Check sheet for the drawn part. Datum: minimum x, y, z corner. Units: mm. A direction names the side the tool comes from. Give positions to 0.01 mm unless a question says otherwise; leave off trailing zeros. Order: outer loops, then holes, each group sorted by start corner. A loop starts at its lowest first (then second) coordinate and runs counter-clockwise, first axis right, second up.
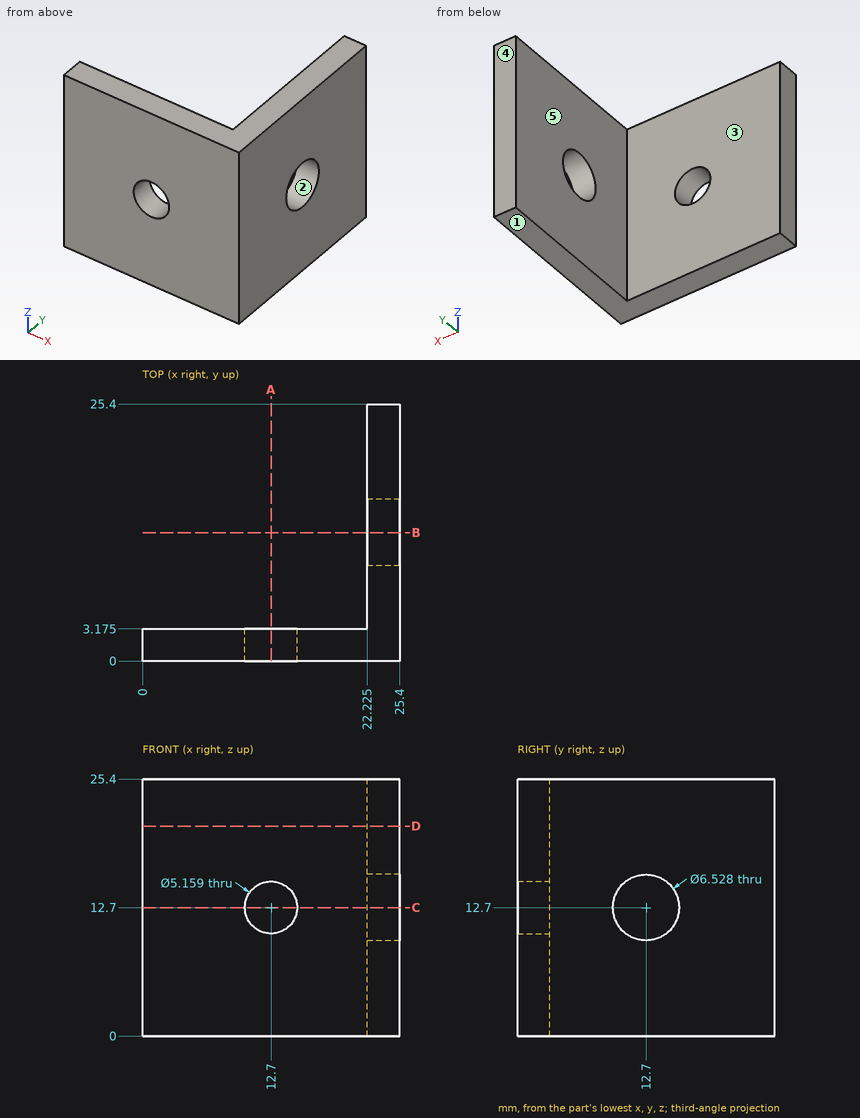
Item 1: Draft check along Z on the marked faces 1, 2 and 3. Enter one of: released by +Z, released by -Z, zero draft, split by the parting line, or undercut.
Reported:
face 1: released by -Z
face 2: undercut
face 3: zero draft
Item 2: Set-up check for the marked faces 4 and 5: record each of +Z, -Z, +X, -X, +Y, -Y from which the full face is reachable in a straight line by a thin tool's end or side.
Reported:
face 4: +Z, -Z, +X, -X, +Y
face 5: +Z, -Z, -X, +Y
Item 3: Sectioned sample at A-A (x = 12.7). Enter the section's corners in (y, z) (1 decimal).
Reported:
outline: (0, 0) - (3.2, 0) - (3.2, 10.1) - (0, 10.1) - close; (0, 15.3) - (3.2, 15.3) - (3.2, 25.4) - (0, 25.4) - close
Item 4: Sectioned sample at B-B (y = 12.7). Enter the section's corners in (x, z) (1 decimal).
Reported:
outline: (22.2, 0) - (25.4, 0) - (25.4, 9.4) - (22.2, 9.4) - close; (22.2, 16) - (25.4, 16) - (25.4, 25.4) - (22.2, 25.4) - close
Item 5: Sectioned sample at C-C (z = 12.7). Enter the section's corners in (x, y) (1 decimal).
Reported:
outline: (0, 0) - (10.1, 0) - (10.1, 3.2) - (0, 3.2) - close; (15.3, 0) - (25.4, 0) - (25.4, 9.4) - (22.2, 9.4) - (22.2, 3.2) - (15.3, 3.2) - close; (22.2, 16) - (25.4, 16) - (25.4, 25.4) - (22.2, 25.4) - close
Item 6: Scan lines: L1, parallel to Z at x = 12.7, y = 1.4; L2, parallel to Y at x = 24.65, z = 12.7. Record each from-to range of solid material in increasing order.
Reported:
L1: z = 0 to 10.12, 15.28 to 25.4
L2: y = 0 to 9.44, 15.96 to 25.4
Item 7: Sectioned sample at D-D (z = 20.75). Enter the section's corners in (x, y) (1 decimal).
Reported:
outline: (0, 0) - (25.4, 0) - (25.4, 25.4) - (22.2, 25.4) - (22.2, 3.2) - (0, 3.2) - close
Item 8: Gauge pin test, flat ends, axial feed: pin 1 (5 mm diameter, centred on x = 3, z = 4.5, fed in from +Y) (3 decimals); pin 2 (11 mm diameter, centred on y = 12, z = 15, fed in from -X) (3 decimals). Record the tip position at first contact, or that the pin passes through.
Reported:
pin 1: stops at y = 3.175
pin 2: stops at x = 22.225
